Here's the drawing with two shaded views (mm, measured from the low corner). I have some questions. Round coordinates to 2 decimals unless told otherwise and drop trailing zeros. Write each loop counter-clockwise with the first axis right and the second up, starting at its lowest first coordinate (ties: lowest second). Pieces come first, ordered by that corner, then holes. Notation, with made-up numbers: M 49.5,-35 L 74.5,-35 A13 cw 74.5,-27 Z; hole C 32.25,57 d6. An arc over 180 degrees is marked long. Answer as a JSON object with one key per item and string values. Group by question number.
1) Please list where this line runs through material, in increasing order: L1, parallel to Z at x = 27.05, y = 1.95. Write a range as [from, to].
2) Suppose I cut it at A-A, the plane z = 34. Write out the boundary of the cut face in (x, y), and give its area (4 significant figures).
3) Suppose I cut it at B-B, the plane y = 0.9. Write out the boundary of the cut face in (x, z), and give its area (3 significant figures).
4) Suppose I cut it at C-C, the plane x = 7.05. Write out the boundary of the cut face in (y, z), and give its area (3 significant figures).
5) If we mould it in two halves opening along X, with no side actions, what happens to the marked faces 1 and 2? For each: +X half, -X half, draft (parallel to the pull), parting line (faces both ways), or undercut.
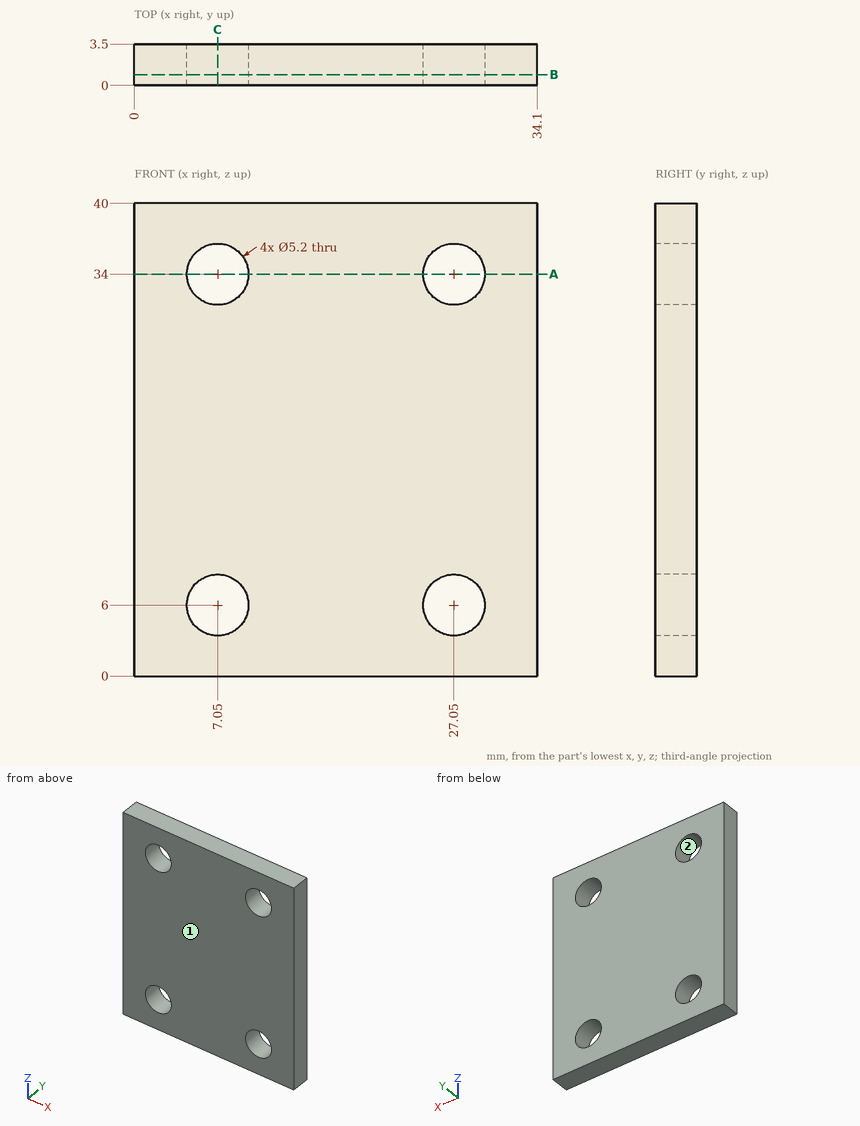
Results:
{
 "1": {"L1": "[0, 3.4], [8.6, 31.4], [36.6, 40]"},
 "2": {"outline": "M 0,0 L 4.45,0 L 4.45,3.5 L 0,3.5 Z; M 9.65,0 L 24.45,0 L 24.45,3.5 L 9.65,3.5 Z; M 29.65,0 L 34.1,0 L 34.1,3.5 L 29.65,3.5 Z", "area": "82.95 mm^2"},
 "3": {"outline": "M 0,0 L 34.1,0 L 34.1,40 L 0,40 Z; hole C 7.05,6 d5.2; hole C 7.05,34 d5.2; hole C 27.05,6 d5.2; hole C 27.05,34 d5.2", "area": "1,280 mm^2"},
 "4": {"outline": "M 0,0 L 3.5,0 L 3.5,3.4 L 0,3.4 Z; M 0,8.6 L 3.5,8.6 L 3.5,31.4 L 0,31.4 Z; M 0,36.6 L 3.5,36.6 L 3.5,40 L 0,40 Z", "area": "104 mm^2"},
 "5": {"face 1": "draft", "face 2": "undercut"}
}
